```python
from build123d import *

# Parameters (mm, degrees)
F1_DEPTH = 25.4


with BuildPart() as f1:
    # F0 (on Front) → F1 (new body)
    with BuildSketch(Plane.XZ):
        with BuildLine():
            ThreePointArc((0, 22.537658), (-0.083312, 20.793829), (0, 19.05))
            Line((0, 19.05), (0, 22.537658))
        make_face()
        with BuildLine():
            Line((0, 19.05), (0, 0))
            Line((0, 0), (69.509163, 0))
            Line((69.509163, 0), (69.509163, 15.319245))
            ThreePointArc((69.509163, 15.319245), (53.830644, 22.622581), (46.110269, 38.1))
            Line((46.110269, 38.1), (12.284626, 38.1))
            ThreePointArc((12.284626, 38.1), (3.850977, 32.127568), (0, 22.537658))
            Line((0, 22.537658), (0, 19.05))
        make_face()
    extrude(amount=F1_DEPTH)


solid = f1.part
```
Part model, mm, in its own coordinate system. A direction names the side the tool comes from. Give positions to 0.01 mm unless a question says otherwise; leave off trailing zeros. Order: outer loops, then holes, each group sorted by start corner. A loop starts at its lowest first (then second) coordinate and runs counter-clockwise, first axis right, second up. Notation, with made-up numbers: (27, -36) - (37, -36) arc R26 ccw to (37, 0) - close; hole circle Ø1 at (24.5, 3). An arc over 180 degrees is marked (long way). Use one line per item in the form item = value.
Item 1: Slice it at A-A on y = -5. Give the cut face in (x, z).
Solution:
outline = (0, 0) - (69.51, 0) - (69.51, 15.32) arc R26.22 cw to (46.11, 38.1) - (12.28, 38.1) arc R18.29 ccw to (0, 22.54) arc R18.29 ccw to (0, 19.05) - close
Item 2: Probe probe 1 along X at (y, z) = (-21.75, 7.5); probe 2 along X at (y, z) = (-23.25, 30); probe 3 along Z at (x, y) = (58.5, -18). List the from-to ranges inside material, lowest first. Write a range as from..to.
Solution:
probe_1 = 0..69.51
probe_2 = 2.4..48.51
probe_3 = 0..19.01
Item 3: Pin check, flat tips, straight feed: pin 1 Ø6 at (y, z) = (-3, 27.5) entering from +X; pin 2 Ø9.5 at (y, z) = (-17, 12) entering from -X; pin 3 Ø6 at (y, z) = (-7.5, 29) entering from -X. Stop position of each tip, or through.
Solution:
pin_1 = 52.08
pin_2 = 0
pin_3 = 0.67
Item 4: Slice it at C-C on x = 53. Give the cut face in (y, z).
Solution:
outline = (-25.4, 0) - (0, 0) - (0, 23.47) - (-25.4, 23.47) - close
Item 5: Which spindle directions (+Z, -Z, +X, -X, +Y, -Y) get a long thin tool onto all of the face, cutting with end or side? Do faces 1 (the face through (3.94, -12.52, 32.24)), 2 (the face through (0, -13, 10)). Say none if no direction does.
Solution:
face_1 = +Z, -X, +Y, -Y
face_2 = -Z, -X, +Y, -Y
Item 6: Slice it at B-B on z = 33. Give the cut face in (x, y).
Solution:
outline = (4.58, -25.4) - (47.29, -25.4) - (47.29, 0) - (4.58, 0) - close
